Could you check a few things on this model? Use its own coordinates, in mm. Coordinates: 2 decimals unless noted, no trailing zeros. Order: outer loops, then holes, each group sorted by start corner. A loop starts at its lowest first (then second) coordinate and runs counter-clockwise, first axis right, second up. Notation, with made-up numbers: (39, -14) - (79, -14) arc R28 ccw to (79, 5) - close; hole circle Ø4 at (-17.5, -12.75). An arc over 180 degrees is marked (long way). Answer as CSV lines item,"result". Start each with the question number.
1. I want a section at A-A, the plane x = -17.5. List the corners of the cut face in (y, z) for me.
2. I want a section at B-B, the plane y = 37.5. List the corners of the cut face in (x, z) for me, and give its area (3 significant figures).
3. I need wall thicknesses on probe 1 along Z at (x, y) = (-7, 30); probe 2 along Z at (x, y) = (18.5, 17); probe 3 along X at (y, z) = (17, 0). Which ranges of each line are inside material? Lowest first, please.
4. For pin 1 (10 mm diameter, centred on y = 29, z = 8, fed in from +X); pin 2 (1 mm diameter, centred on y = 27, z = -2.5, fed in from -X); pin 3 (2 mm diameter, centred on x = 2, y = 33.5, fed in from +Z), each with a flat end and sliding along its axis, tell me the tip position at first contact or that it passes through.
from build123d import *

# Parameters (mm, degrees)
BOSS_EXTRU_1_DEPTH = 50
D_POUILLE7_ANGLE   = 15
D_POUILLE8_ANGLE   = -15


with BuildPart() as part:
    # Esquisse1 → Boss.-Extru.1 (new body)
    with BuildSketch(Plane(origin=(0, 0, 0), x_dir=(1, 0, 0), z_dir=(0, 1, 0))):
        Polygon((25.259584223, 24.737691987), (-24.737691987, 25.259584223), (-25.259584223, -24.737691987), (24.737691987, -25.259584223), align=None)
    extrude(amount=BOSS_EXTRU_1_DEPTH)

    # Dépouille7
    d_pouille7_faces = [part.faces().sort_by_distance(p)[0] for p in [
        (0.260946118, 25, -24.998638105),
        (-0.260946118, 25, 24.998638105),
    ]]
    draft(d_pouille7_faces, Plane(origin=(-24.737691987, 50, -25.259584223), x_dir=(0.010437844720406831, 0, -0.9999455242149908), z_dir=(-0.9999455242149908, 0, -0.010437844720406831)), D_POUILLE7_ANGLE)

    # Dépouille8
    d_pouille8_faces = [part.faces().sort_by_distance(p)[0] for p in [
        (0.33086642, 25, -31.697002998),
        (-0.33086642, 25, 31.697002998),
    ]]
    draft(d_pouille8_faces, Plane(origin=(-24.737691987, 50, -25.259584223), x_dir=(0.010437844720406831, 0, -0.9999455242149908), z_dir=(-0.9999455242149908, 0, -0.010437844720406831)), D_POUILLE8_ANGLE)


solid = part.part
Solved:
1,outline,"(0, -23.24) - (50, -23.24) - (50, 22.75) - (0, 22.75) - close"
2,outline,"(-25.26, 24.74) - (-24.74, -25.26) - (25.12, -11.34) - (24.88, 11.86) - close"
2,area,"1,830 mm2"
3,probe 1,"z = -20.31 to 20.05"
3,probe 2,"z = -13.19 to 13.5"
3,probe 3,"x = -25 to 25"
4,pin 1,"stops at x = 24.97"
4,pin 2,"stops at x = -24.98"
4,pin 3,"stops at z = 17.99"
